```python
from build123d import *

# Parameters (mm, degrees)
BOSS_EXTRUDE1_DEPTH = 100
CUT_EXTRUDE1_DEPTH  = 101
FILLET1_R           = 0.25


with BuildPart() as part:
    # Sketch2 → Boss-Extrude1 (new body)
    with BuildSketch(Plane.XY):
        with BuildLine():
            Line((-38.157568057, -12), (38.157568057, -12))
            ThreePointArc((38.157568057, -12), (0, -40), (-38.157568057, -12))
        make_face()
    extrude(amount=BOSS_EXTRUDE1_DEPTH)

    # Sketch3 → Cut-Extrude1 (cut, through all)
    with BuildSketch(Plane(origin=(0, 0, 0), x_dir=(-1, 0, 0), z_dir=(0, 0, -1))):
        Polygon((-11.07179677, -12), (-18, -24), (18, -24), (11.07179677, -12), align=None)
    extrude(amount=-CUT_EXTRUDE1_DEPTH, mode=Mode.SUBTRACT)

    # Fillet1
    fillet1_edges = [part.edges().sort_by_distance(p)[0] for p in [
        (11.07179677, -12, 50),
        (-11.07179677, -12, 50),
        (-18, -24, 50),
        (18, -24, 50),
    ]]
    fillet(fillet1_edges, radius=FILLET1_R)


solid = part.part
```
Design review of the part built by this model. Coordinates are the model's own, in mm. A direction names the side the tool comes from. Coordinates: 2 decimals unless noted, no trailing zeros. Write each loop counter-clockwise with the first axis right and the second up, starting at its lowest first coordinate (ties: lowest second). Pieces come first, ordered by that corner, then holes. Notation, with made-up numbers: M 4,70.5 L 34,70.5 A21 ccw 34,95.5 Z; hole C 53,50.5 d10. An arc over 180 degrees is marked long. Answer as a JSON object with one key per item and string values.
Item 1: Add section B-B, the plane x = 15.5. Give the boundary of the cut face in (y, z), and give its area (3 significant figures).
Outcome:
{"outline": "M -36.87,0 L -24,0 L -24,100 L -36.87,100 Z; M -19.67,0 L -12,0 L -12,100 L -19.67,100 Z", "area": "2,050 mm²"}
Item 2: Add section D-D, the plane y = -32. Give the boundary of the cut face in (x, z).
Outcome:
{"outline": "M -24,0 L 24,0 L 24,100 L -24,100 Z"}
Item 3: Draft analysis for pull direction Y (two halves, no side actions). For faces 1 (the flat face through (-25, -12, 49)), 2 (the flat face through (14.49, -17.92, 49.3)), 3 (the flat face through (1, -26, 0)), 4 (the cylindrical face through (0.709, -39.994, 49.3)), state which applies: pulls with the +Y half, pulls with the -Y half, needs draft (parallel to the pull), parting line crosses it, or undercut.
Outcome:
{"face 1": "pulls with the +Y half", "face 2": "undercut", "face 3": "needs draft", "face 4": "pulls with the -Y half"}
Item 4: Add section C-C, the plane y = -21. Give the boundary of the cut face in (x, z).
Outcome:
{"outline": "M -34.04,0 L -16.27,0 L -16.27,100 L -34.04,100 Z; M 16.27,0 L 34.04,0 L 34.04,100 L 16.27,100 Z"}
Item 5: Insertion check: pin 1 Ø3 at (y, z) = (-21.5, 28) entering from +X; pin 2 Ø10 at (x, z) = (-24, 55) entering from -Y; pin 3 Ø6 at (y, z) = (-25.5, 82.5) entering from -X. Each pin has a flat end and moves straight along its axis. Give the tip position at first contact, or say it passes through.
Outcome:
{"pin 1": "x = 34.64", "pin 2": "y = -35.2", "pin 3": "x = -33.07"}
Item 6: Wall thickness on probe 1 along X at (y, z) = (-13.5, 5.5); probe 2 along X at (y, z) = (-17.5, 26); probe 3 along Y at (x, z) = (14.5, 11.5): over which ranges is each line inside the solid? List them lowest first.
Outcome:
{"probe 1": "-37.65 to -11.94, 11.94 to 37.65", "probe 2": "-35.97 to -14.25, 14.25 to 35.97", "probe 3": "-37.28 to -24, -17.94 to -12"}
Item 7: Machinability: for faces 5 (the flat face through (0, -24, 49)), 6 (the flat face through (1, -26, 100)), which of the approach directions +Z, -Z, +X, -X, +Y, -Y give a long, thin tool a straight path to every point of the face, cutting with its end or side? Answer none if there is none.
Outcome:
{"face 5": "+Z, -Z", "face 6": "+Z, +X, -X, +Y, -Y"}
